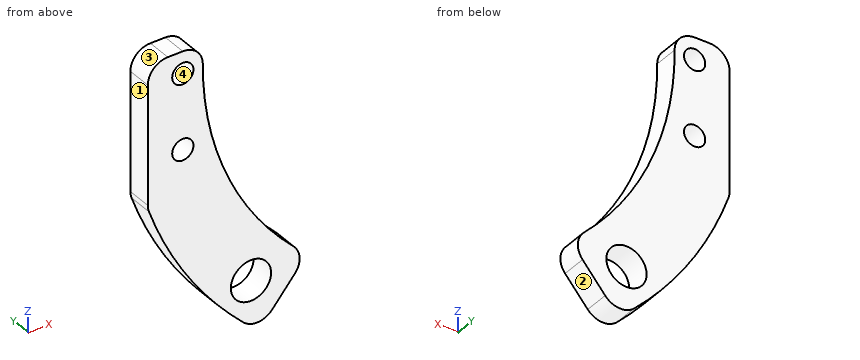
from build123d import *

# Parameters (mm, degrees)
SKETCH1_R               = 4.025
SKETCH1_R_2             = 2.125
BOSS_EXTRUDE1_DEPTH     = 5
SKETCH2_W               = 28.904595792
SKETCH2_H               = 55.332112
CUT_EXTRUDE1_DEPTH      = 1
CUT_EXTRUDE1_DEPTH_BACK = 6
SKETCH3_W               = 24.207106467
SKETCH3_H               = 21.100530829
CUT_EXTRUDE2_DEPTH      = 1
CUT_EXTRUDE2_DEPTH_BACK = 6
FILLET1_R               = 4


with BuildPart() as part:
    # Sketch1 → Boss-Extrude1 (new body)
    with BuildSketch(Plane(origin=(0, 0, 0), x_dir=(1, 0, 0), z_dir=(0, 1, 0))):
        with BuildLine():
            Line((-47.75734818, 56.526415903), (-38.07680463, 45.068358625))
            ThreePointArc((-38.07680463, 45.068358625), (-56.716415256, 16.255714087), (-56.169167779, -18.056151058))
            Line((-56.169167779, -18.056151058), (-70.449464672, -22.646697938))
            ThreePointArc((-70.449464672, -22.646697938), (-71.135842864, 20.388522754), (-47.75734818, 56.526415903))
        make_face()
        with Locations((-49.366374859, 46.034889304)):
            Circle(SKETCH1_R, mode=Mode.SUBTRACT)
        with Locations((-63, 0)):
            Circle(SKETCH1_R_2, mode=Mode.SUBTRACT)
        with Locations((-63, -15)):
            Circle(SKETCH1_R_2, mode=Mode.SUBTRACT)
        with Locations((-63, 15)):
            Circle(SKETCH1_R_2, mode=Mode.SUBTRACT)
    extrude(amount=BOSS_EXTRUDE1_DEPTH)

    # Sketch2 → Cut-Extrude1 (cut, two sides)
    with BuildSketch(Plane(origin=(0, 5, 0), x_dir=(1, 0, 0), z_dir=(0, 1, 0))) as cut_extrude1_sk:
        with Locations((-84.452297896, 0)):
            Rectangle(SKETCH2_W, SKETCH2_H)
    extrude(amount=CUT_EXTRUDE1_DEPTH, mode=Mode.SUBTRACT)
    extrude(cut_extrude1_sk.sketch, amount=-CUT_EXTRUDE1_DEPTH_BACK, mode=Mode.SUBTRACT)

    # Sketch3 → Cut-Extrude2 (cut, two sides)
    with BuildSketch(Plane(origin=(0, 5, 0), x_dir=(1, 0, 0), z_dir=(0, 1, 0))) as cut_extrude2_sk:
        with Locations((-57.896446767, -14.949043558)):
            Rectangle(SKETCH3_W, SKETCH3_H)
    extrude(amount=CUT_EXTRUDE2_DEPTH, mode=Mode.SUBTRACT)
    extrude(cut_extrude2_sk.sketch, amount=-CUT_EXTRUDE2_DEPTH_BACK, mode=Mode.SUBTRACT)

    # Fillet1
    fillet1_edges = [part.edges().sort_by_distance(p)[0] for p in [
        (-70, 2.5, -24),
        (-58.835794809, 2.5, 4.398778143),
        (-70, 2.5, 4.398778143),
        (-47.75734818, 2.5, -56.526415903),
        (-38.07680463, 2.5, -45.068358625),
    ]]
    fillet(fillet1_edges, radius=FILLET1_R)


solid = part.part
Read the model definition and answer for the solid it produces. Units are mm, in the model's axes. Face numbers are marked on the shaded views. Round coordinates to 2 decimals unless told otherwise and drop trailing zeros. Order: outer loops, then holes, each group sorted by start corner. A loop starts at its lowest first (then second) coordinate and runs counter-clockwise, first axis right, second up.
1) The part is cut by section D-D on z = -15. Write down the section's boundary in (x, y) (3 decimals), plus the area to 3 significant figures.
2) The part is cut by section C-C on y = 4. Write down the section's boundary in (x, z) (3 decimals).
3) Straight lines are drawn through the part: L1, parallel to Z at x = -63, y = 2.55 (3 decimals); L2, parallel to Z at x = -64.5, y = 2.65; L3, parallel to X at y = 3.3, z = 0 (3 decimals). For each, find the intervals that lie inside material, in ascending order.
4) The part is cut by section A-A on x = -64.5. Write down the section's boundary in (y, z).
5) The part is cut by section B-B on x = -49. Write down the section's boundary in (y, z), plus the area to 3 significant figures.
6) The mould has two halves that part along Z. Classify the marked faces 1, 2, 3 and 4: released by +Z, released by -Z, zero draft, split by the parting line, or undercut.
7) Flat-ended cylindrical pins translate along their axes: pin 1 (2 mm diameter, centred on y = 2.5, z = -43, fed in from +X); pin 2 (4 mm diameter, centred on x = -63, z = 0, fed in from -Y); pin 3 (1 mm diameter, centred on x = -45, y = 4, fed in from -Z); pin 4 (1 mm diameter, centred on y = 1, z = -6, fed in from +X). Find the tip coordinate at first contact, or state that the pin passes through.
Resolved:
1. outline: (-70, 0) - (-65.125, 0) - (-65.125, 5) - (-70, 5) - close; (-60.875, 0) - (-57.061, 0) - (-57.061, 5) - (-60.875, 5) - close
1. area: 43.4 mm2
2. outline: (-70, -23.324) arc R4 ccw to (-69.771, -24.657) arc R74 ccw to (-50.909, -53.705) arc R4 ccw to (-45.102, -53.384) - (-40.576, -48.027) arc R4 ccw to (-40.861, -42.56) arc R59 cw to (-58.999, 0.373) arc R4 ccw to (-62.999, 4.399) - (-66, 4.399) arc R4 ccw to (-70, 0.399) - close; hole circle Ø4.25 at (-63, -15); hole circle Ø4.25 at (-63, 0); hole circle Ø8.05 at (-49.366, -46.035)
3. L1: z = -38.82 to -17.125, -12.875 to -2.125, 2.125 to 4.399
3. L2: z = -36.27 to -16.51, -13.49 to -1.51, 1.51 to 4.4
3. L3: x = -70 to -65.125, -60.875 to -59
4. outline: (0, -36.27) - (5, -36.27) - (5, -16.51) - (0, -16.51) - close; (0, -13.49) - (5, -13.49) - (5, -1.51) - (0, -1.51) - close; (0, 1.51) - (5, 1.51) - (5, 4.4) - (0, 4.4) - close
5. outline: (0, -54.71) - (5, -54.71) - (5, -50.04) - (0, -50.04) - close; (0, -42.03) - (5, -42.03) - (5, -32.86) - (0, -32.86) - close
5. area: 69.2 mm2
6. face 1: zero draft
6. face 2: released by -Z
6. face 3: released by +Z
6. face 4: undercut
7. pin 1: stops at x = -39.9
7. pin 2: passes through
7. pin 3: stops at z = -53.79
7. pin 4: stops at x = -58.64
